Autodesk Inventor part; units mm, degrees
ref_plane "YZ Plane" through (0, 0, 0) normal (1, 0, 0) x (0, 1, 0)
ref_plane "XZ Plane" through (0, 0, 0) normal (0, 1, 0) x (-1, 0, 0)
ref_plane "XY Plane" through (0, 0, 0) normal (0, 0, 1) x (1, 0, 0)
sketch "Esboço1" plane through (0, 0, 0) normal (0, 0, 1) x (1, 0, 0)
  circle A0 centre (0, 0) radius 12.3
  dimension "d0" = 24.6
extrude "Extrusão1" add sketch "Esboço1" along normal blind 1.5
sketch "Esboço2" plane through (0, 0, 1.5) normal (0, 0, 1) x (1, 0, 0)
  circle A0 centre (0, 0) radius 7
  dimension "d3" = 14
extrude "Extrusão2" add sketch "Esboço2" along normal blind 5
sketch "Esboço3" plane through (0, 0, 6.5) normal (0, 0, 1) x (1, 0, 0)
  circle A0 centre (0, 0) radius 9.25
  dimension "d6" = 18.5
extrude "Extrusão3" add sketch "Esboço3" along normal blind 1.5
sketch "Esboço4" plane through (0, 0, 8) normal (0, 0, 1) x (1, 0, 0)
  circle A0 centre (0, 0) radius 7.5
  dimension "d9" = 15
extrude "Extrusão4" add sketch "Esboço4" along normal blind 3
sketch "Esboço5" plane through (0, 0, 11) normal (0, 0, 1) x (1, 0, 0)
  circle A0 centre (0, 0) radius 9
  dimension "d12" = 18
extrude "Extrusão5" add sketch "Esboço5" along normal blind 1
sketch "Esboço6" plane through (0, 0, 12) normal (0, 0, 1) x (1, 0, 0)
  circle A0 centre (0, 0) radius 7.5
  dimension "d15" = 15
extrude "Extrusão6" add sketch "Esboço6" along normal blind 2
sketch "Esboço7" plane through (0, 0, 14) normal (0, 0, 1) x (1, 0, 0)
  circle A0 centre (0, 0) radius 7
  dimension "d18" = 14
extrude "Extrusão7" add sketch "Esboço7" along normal blind 9
chamfer "Chanfro1" distance 0.5 angle 45 1 edges at (-7, 0, 14)
sketch "Esboço8" plane through (0, 0, 23) normal (0, 0, 1) x (1, 0, 0)
  circle A0 centre (0, 0) radius 6
  dimension "d24" = 12
extrude "Extrusão8" cut sketch "Esboço8" against normal blind 22
properties part number "BOTÃO"
Verification items for the finished model (mm, model axes). A direction names the side the tool comes from. Round coordinates to 2 decimals unless told otherwise and drop trailing zeros. Order: outer loops, then holes, each group sorted by start corner. A loop starts at its lowest first (then second) coordinate and runs counter-clockwise, first axis right, second up.
1. Section check D-D on x = -8. Record the cut outline in (y, z), then the cut area to 3 significant figures.
Final values:
outline: (-9.34, 0) - (9.34, 0) - (9.34, 1.5) - (-9.34, 1.5) - close; (-4.64, 6.5) - (4.64, 6.5) - (4.64, 8) - (-4.64, 8) - close; (-4.12, 11) - (4.12, 11) - (4.12, 12) - (-4.12, 12) - close
area: 50.2 mm2
2. Release check for a two-part mould opening along X. For faces 1 (the flat face through (-7, 2, 6.5)), 2 (the cylindrical face through (-6, 0, 12)), 3 (the cylindrical face through (-2.7, 12, 0.7)) record: +X half, -X half, draft (parallel to the pull), parting line (faces both ways), or undercut.
Final values:
face 1: draft
face 2: undercut
face 3: parting line
3. Thickness scan on L1, parallel to Z at x = 7.5, y = 0.75; L2, parallel to Z at x = -5.25, y = 2.25; L3, parallel to X at y = 4.75, z = 3.75. Record the ranges inside material, lowest first.
Final values:
L1: z = 0 to 1.5, 6.5 to 8, 11 to 12
L2: z = 0 to 1
L3: x = -5.14 to -3.67, 3.67 to 5.14
4. Access from +Z, -Z, +X, -X, +Y, -Y to the whole of each face (thin tool, end or side, straight path). Record for faces 4 (the cylindrical face through (-7.493, -0.33, 9.479)), 5 (the flat face through (6, 2, 23)), 6 (the cylindrical face through (-1.172, -8.923, 11.493)).
Final values:
face 4: none
face 5: +Z, +X, -X, +Y, -Y
face 6: +Z
5. Go/stop test with flat-tipped pins: P1, Ø4, axis at y = 3.5, z = 18.5, coming from the +X side; P2, Ø1, axis at y = 2, z = 18.5, coming from the -X side; P3, Ø4, axis at y = 6.5, z = 18, coming from the +X side. Record where each tip stops, or that it passes through.
Final values:
P1: stops at x = 6.84
P2: stops at x = -6.84
P3: stops at x = 5.36
6. Section check C-C on z = 19.75. Record the cut outline in (x, y), then the cut area to 3 significant figures.
Final values:
outline: circle Ø14 at (0, 0); hole circle Ø12 at (0, 0)
area: 40.8 mm2
